Check sheet for the modelled part. Datum: model origin and axes. Units: mm. Coordinates: 2 decimals unless noted, no trailing zeros. Loops run counter-clockwise (first coordinate to the right, second up) from the corner with the lowest first, then second, coordinate; pieces in that order, holes last. Notation, with made-up numbers: (-9.75, 42.5) -> (3.25, 42.5) arc R24 cw to (3.25, 63.5) -> close; hole circle Ø11 at (-1.75, 79.5). An arc over 180 degrees is marked (long way). Use CSV: the item, a comma, the result in double quotes. Start each with the question number.
1. Sectioned sample at B-B, the plane x = -39. Record the cut outline in (y, z), and give its area (3 significant figures).
2. Sectioned sample at A-A, the plane y = -34. Record the cut outline in (x, z).
3. Gauge pin test, flat ends, axial feed: pin 1 (3 mm diameter, centred on x = -21, y = 38.5, fed in from -Z); pin 2 (4 mm diameter, centred on y = -2, z = 246.5, fed in from -X); pin 3 (1 mm diameter, centred on x = -1, z = 213, fed in from -Y). Record the tip position at first contact, or that the pin passes through.
4. Thickness scan on L1, parallel to X at y = 12.5, z = 391.5; L2, parallel to Z at x = -5.5, y = -45; L3, parallel to Z at x = -3, y = -12.5. Record the ranges inside material, lowest first.
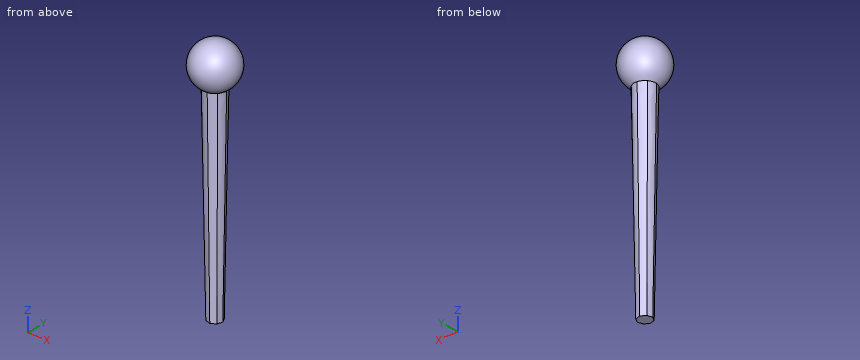
```python
from build123d import *


# Not quite as in the source:
# - the arcs of a loft's sections are written as splines that run evenly, so that the points pair up as in the source's solid


with BuildPart() as f3:
    # F2 (on offset) → F3 section 0
    with BuildSketch(Plane.XY.offset(500)):
        with BuildLine():
            add(Edge.make_bspline(
                [(3.1036920521, -24.8065937937), (4.7272798193, -24.6034576239), (6.3308207683, -24.2404209935), (9.4363429336, -23.2084625424), (10.9382473598, -22.5395662389), (13.782772681, -20.9215792608), (15.1253232396, -19.972528594), (17.5995382038, -17.8306914211), (18.7311414296, -16.6379578761), (19.7355523864, -15.3462689929)],
                knots=[0, 0, 0, 0, 0.25, 0.25, 0.5, 0.5, 0.75, 0.75, 1, 1, 1, 1], degree=3))
            add(Edge.make_bspline(
                [(19.7355523864, -15.3462689929), (20.7399633433, -14.0545801097), (21.617132359, -12.6639997676), (23.0833633226, -9.7383591666), (23.6723890149, -8.2033712501), (24.5396825947, -5.0478985421), (24.8179290366, -3.427491776), (25.0529556268, -0.1634500075), (25.0097299635, 1.480104285), (24.8065937937, 3.1036920521)],
                knots=[0, 0, 0, 0, 0.25, 0.25, 0.5, 0.5, 0.75, 0.75, 1, 1, 1, 1], degree=3))
            add(Edge.make_bspline(
                [(24.8065937937, 3.1036920521), (24.6034576239, 4.7272798193), (24.2404209935, 6.3308207683), (23.2084625424, 9.4363429336), (22.5395662389, 10.9382473598), (20.9215792608, 13.782772681), (19.972528594, 15.1253232396), (17.8306914211, 17.5995382038), (16.6379578761, 18.7311414296), (15.3462689929, 19.7355523864)],
                knots=[0, 0, 0, 0, 0.25, 0.25, 0.5, 0.5, 0.75, 0.75, 1, 1, 1, 1], degree=3))
            add(Edge.make_bspline(
                [(15.3462689929, 19.7355523864), (14.0545801097, 20.7399633433), (12.6639997676, 21.617132359), (9.7383591666, 23.0833633226), (8.2033712501, 23.6723890149), (5.0478985421, 24.5396825947), (3.427491776, 24.8179290366), (0.1634500075, 25.0529556268), (-1.480104285, 25.0097299635), (-3.1036920521, 24.8065937937)],
                knots=[0, 0, 0, 0, 0.25, 0.25, 0.5, 0.5, 0.75, 0.75, 1, 1, 1, 1], degree=3))
            add(Edge.make_bspline(
                [(-3.1036920521, 24.8065937937), (-4.7272798193, 24.6034576239), (-6.3308207683, 24.2404209935), (-9.4363429336, 23.2084625424), (-10.9382473598, 22.5395662389), (-13.782772681, 20.9215792608), (-15.1253232396, 19.972528594), (-17.5995382038, 17.8306914211), (-18.7311414296, 16.6379578761), (-19.7355523864, 15.3462689929)],
                knots=[0, 0, 0, 0, 0.25, 0.25, 0.5, 0.5, 0.75, 0.75, 1, 1, 1, 1], degree=3))
            add(Edge.make_bspline(
                [(-19.7355523864, 15.3462689929), (-20.7399633433, 14.0545801097), (-21.617132359, 12.6639997676), (-23.0833633226, 9.7383591666), (-23.6723890149, 8.2033712501), (-24.5396825947, 5.0478985421), (-24.8179290366, 3.427491776), (-25.0529556268, 0.1634500075), (-25.0097299635, -1.480104285), (-24.8065937937, -3.1036920521)],
                knots=[0, 0, 0, 0, 0.25, 0.25, 0.5, 0.5, 0.75, 0.75, 1, 1, 1, 1], degree=3))
            add(Edge.make_bspline(
                [(-24.8065937937, -3.1036920521), (-24.6034576239, -4.7272798193), (-24.2404209935, -6.3308207683), (-23.2084625424, -9.4363429336), (-22.5395662389, -10.9382473598), (-20.9215792608, -13.782772681), (-19.972528594, -15.1253232396), (-17.8306914211, -17.5995382038), (-16.6379578761, -18.7311414296), (-15.3462689929, -19.7355523864)],
                knots=[0, 0, 0, 0, 0.25, 0.25, 0.5, 0.5, 0.75, 0.75, 1, 1, 1, 1], degree=3))
            add(Edge.make_bspline(
                [(-15.3462689929, -19.7355523864), (-14.0545801097, -20.7399633433), (-12.6639997676, -21.617132359), (-9.7383591666, -23.0833633226), (-8.2033712501, -23.6723890149), (-5.0478985421, -24.5396825947), (-3.427491776, -24.8179290366), (-0.1634500075, -25.0529556268), (1.480104285, -25.0097299635), (3.1036920521, -24.8065937937)],
                knots=[0, 0, 0, 0, 0.25, 0.25, 0.5, 0.5, 0.75, 0.75, 1, 1, 1, 1], degree=3))
        make_face()
    # F1 (on Top) → F3 section 1
    with BuildSketch(Plane.XY):
        Polygon((2.0156472416, -16.1102781829), (12.8169647829, -9.9664091169), (16.1102781829, 2.0156472416), (9.9664091169, 12.8169647829), (-2.0156472416, 16.1102781829), (-12.8169647829, 9.9664091169), (-16.1102781829, -2.0156472416), (-9.9664091169, -12.8169647829), align=None)
    loft(ruled=True)

    # F5 (on offset) → F6 (revolve)
    with BuildSketch(Plane.XY.offset(500)):
        with BuildLine():
            Line((0, -50), (0, 50))
            ThreePointArc((0, 50), (-50, 0), (0, -50))
        make_face()
    revolve(axis=Axis((0, 0, 500), (0, -1, 0)))


solid = f3.part
```
Completed:
1,outline,"circle Ø62.58 at (0, 500)"
1,area,"3,080 mm²"
2,outline,"circle Ø73.32 at (0, 500)"
3,pin 1,"z = 473.43"
3,pin 2,"x = -20.43"
3,pin 3,"y = -19.52"
4,L1,"-19.3 to 19.11"
4,L2,"478.91 to 521.09"
4,L3,"0 to 548.32"
